Geometry check sheet. Reference: drawing and pictorial views, mm from the part's lowest x, y, z. A direction names the side the tool comes from. Coordinates: 2 decimals unless noted, no trailing zeros. Loops run counter-clockwise (first coordinate to the right, second up) from the corner with the lowest first, then second, coordinate; pieces in that order, holes last. Notation, with made-up numbers: (-28.75, 56) -> (23.25, 56) arc R29 ccw to (23.25, 84) -> close; hole circle Ø1 at (10.5, 23.5). An arc over 180 degrees is marked (long way). Answer as a JSON object with one key per item and string values. Group by question number.
Q1. Cross-section at D-D on y = 204. Record the boundary of the cut face in (x, z).
Q2. Set-up check for the marked faces 1 and 2: record each of +Z, -Z, +X, -X, +Y, -Y from which the full face is reachable in a straight line by a thin tool's end or side.
Q3. Gauge pin test, flat ends, axial feed: pin 1 Ø1.5 at (y, z) = (76.5, 27) entering from +X; pin 2 Ø1.5 at (x, y) = (191.5, 279) entering from -Z; pin 3 Ø5 at (x, y) = (242.5, 301.5) entering from +Z. Record the tip position at first contact, or that the pin passes through.
Q4. Cross-section at C-C on x = 213.29. Record the boundary of the cut face in (y, z) (3 decimals).
Q5. Cross-section at A-A on x = 300. Record the boundary of the cut face in (y, z).
Q6. Scan lines: L1, parallel to Y at x = 300, z = 6; L2, parallel to Z at x = 204, y = 387.5; L3, parallel to Y at x = 289, z = 5.5. Record each from-to range of solid material in increasing order.
Q7. Cross-section at B-B on y = 400. Record the boundary of the cut face in (x, z).
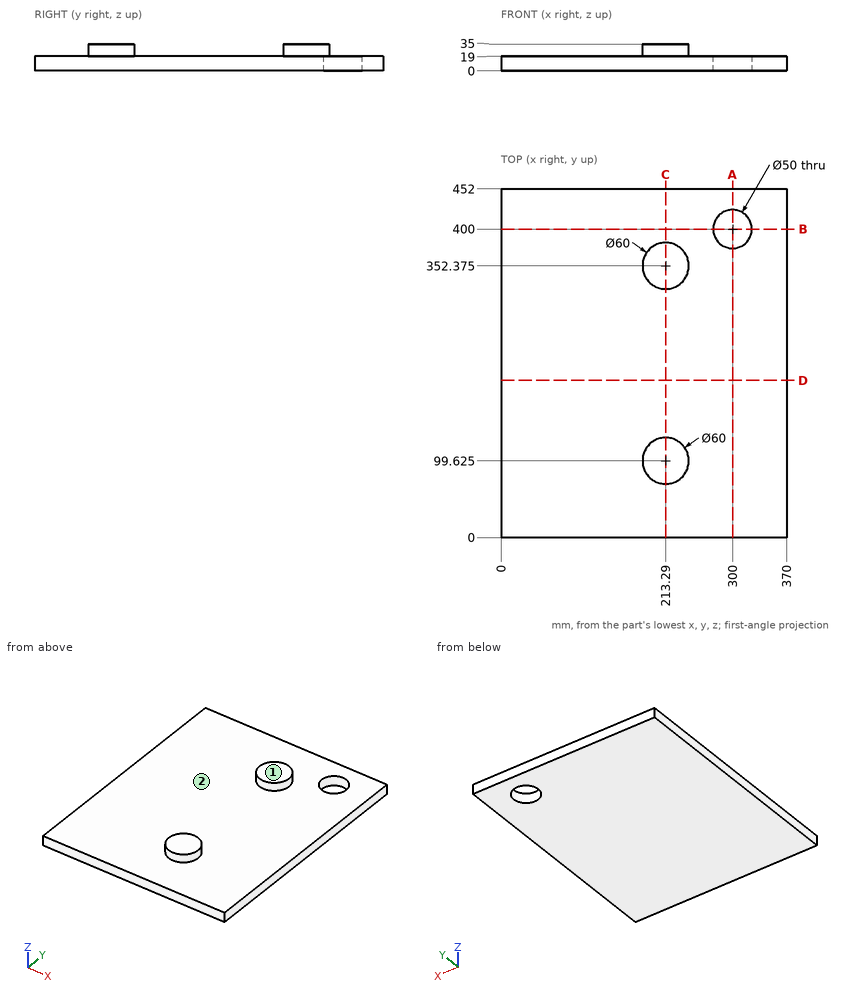
Computed values:
{
 "1": {"outline": "(0, 0) -> (370, 0) -> (370, 19) -> (0, 19) -> close"},
 "2": {"face 1": "+Z, +X, -X, +Y, -Y", "face 2": "+Z"},
 "3": {"pin 1": "stops at x = 233.27", "pin 2": "stops at z = 0", "pin 3": "stops at z = 19"},
 "4": {"outline": "(0, 0) -> (452, 0) -> (452, 19) -> (382.375, 19) -> (382.375, 35) -> (322.375, 35) -> (322.375, 19) -> (129.625, 19) -> (129.625, 35) -> (69.625, 35) -> (69.625, 19) -> (0, 19) -> close"},
 "5": {"outline": "(0, 0) -> (375, 0) -> (375, 19) -> (0, 19) -> close; (425, 0) -> (452, 0) -> (452, 19) -> (425, 19) -> close"},
 "6": {"L1": "y = 0 to 375, 425 to 452", "L2": "z = 0 to 19", "L3": "y = 0 to 377.55, 422.45 to 452"},
 "7": {"outline": "(0, 0) -> (275, 0) -> (275, 19) -> (0, 19) -> close; (325, 0) -> (370, 0) -> (370, 19) -> (325, 19) -> close"}
}
